```python
from build123d import *

# Parameters (mm, degrees)
SKETCH_1_W               = 72
SKETCH_1_H               = 100
EXTRUDE_1_DEPTH          = 5
SKETCH_2_W               = 72
SKETCH_2_H               = 5
EXTRUDE_2_DEPTH          = 24
CUT_EXTRUDE_1_DEPTH      = 83.443920334
CUT_EXTRUDE_1_DEPTH_BACK = 83.443920334
SKETCH_3_W               = 3
SKETCH_3_H               = 50
CUT_EXTRUDE_2_DEPTH      = 83.443920334
CUT_EXTRUDE_2_DEPTH_BACK = 83.443920334
SKETCH_5_R               = 1.75
CUT_EXTRUDE_3_DEPTH      = 83.443920334
CUT_EXTRUDE_3_DEPTH_BACK = 83.443920334
SKETCH_6_R               = 1.75
CUT_EXTRUDE_4_DEPTH      = 83.443920334
CUT_EXTRUDE_4_DEPTH_BACK = 83.443920334
SKETCH_7_W               = 24
SKETCH_7_H               = 12
FILLET_1_R               = 5
FILLET_2_R               = 2
CUT_EXTRUDE_5_DEPTH      = 83.443920334
CUT_EXTRUDE_5_DEPTH_BACK = 83.443920334
SKETCH_8_R               = 1.75


with BuildPart() as part:
    # 草图1 → 凸台-拉伸1 (new body)
    with BuildSketch(Plane(origin=(0, 0, 0), x_dir=(1, 0, 0), z_dir=(0, 1, 0))):
        Rectangle(SKETCH_1_W, SKETCH_1_H)
    extrude(amount=EXTRUDE_1_DEPTH)

    # 草图2 → 凸台-拉伸2 (add)
    with BuildSketch(Plane.XY.offset(50)):
        with Locations((0, 2.5)):
            Rectangle(SKETCH_2_W, SKETCH_2_H)
    extrude(amount=EXTRUDE_2_DEPTH)

    # 草图3 → 切除-拉伸1 (cut, two sides: drawn at the far end of the back side and taken through both)
    with BuildSketch(Plane(origin=(0, 5, 0), x_dir=(1, 0, 0), z_dir=(0, 1, 0)).offset(-CUT_EXTRUDE_1_DEPTH_BACK)):
        with Locations((-34.5, 25)):
            Rectangle(SKETCH_3_W, SKETCH_3_H)
        with Locations((34.5, 25)):
            Rectangle(SKETCH_3_W, SKETCH_3_H)
        with Locations((-34.5, -49)):
            Rectangle(SKETCH_3_W, SKETCH_3_H)
        with Locations((34.5, -49)):
            Rectangle(SKETCH_3_W, SKETCH_3_H)
    extrude(amount=CUT_EXTRUDE_1_DEPTH + CUT_EXTRUDE_1_DEPTH_BACK, mode=Mode.SUBTRACT)

    # 草图5 → 切除-拉伸2 (cut, two sides: drawn at the far end of the back side and taken through both)
    with BuildSketch(Plane(origin=(0, 5, 0), x_dir=(1, 0, 0), z_dir=(0, 1, 0)).offset(-CUT_EXTRUDE_2_DEPTH_BACK)):
        with Locations(Location((-23.5, 40.5, 0), (0, 0, 270))):
            Circle(SKETCH_5_R)
    extrude(amount=CUT_EXTRUDE_2_DEPTH + CUT_EXTRUDE_2_DEPTH_BACK, mode=Mode.SUBTRACT)

    # 草图6 → 切除-拉伸3 (cut, two sides: drawn at the far end of the back side and taken through both)
    with BuildSketch(Plane(origin=(0, 5, 0), x_dir=(1, 0, 0), z_dir=(0, 1, 0)).offset(-CUT_EXTRUDE_3_DEPTH_BACK)):
        with Locations(Location((23.5, 40.5, 0), (0, 0, 270))):
            Circle(SKETCH_6_R)
        with Locations(Location((-23.5, -64.5, 0), (0, 0, 270))):
            Circle(SKETCH_6_R)
        with Locations(Location((23.5, -64.5, 0), (0, 0, 270))):
            Circle(SKETCH_6_R)
    extrude(amount=CUT_EXTRUDE_3_DEPTH + CUT_EXTRUDE_3_DEPTH_BACK, mode=Mode.SUBTRACT)

    # 草图7 → 切除-拉伸4 (cut, two sides: drawn at the far end of the back side and taken through both)
    with BuildSketch(Plane(origin=(0, 5, 0), x_dir=(1, 0, 0), z_dir=(0, 1, 0)).offset(-CUT_EXTRUDE_4_DEPTH_BACK)):
        with Locations((0, -50)):
            Rectangle(SKETCH_7_W, SKETCH_7_H)
        with Locations((0, 26)):
            Rectangle(SKETCH_7_W, SKETCH_7_H)
    extrude(amount=CUT_EXTRUDE_4_DEPTH + CUT_EXTRUDE_4_DEPTH_BACK, mode=Mode.SUBTRACT)

    # 圆角1
    fillet_1_edges = [part.edges().sort_by_distance(p)[0] for p in [
        (33, 2.5, -50),
        (-33, 2.5, 74),
        (33, 2.5, 74),
        (-33, 2.5, -50),
    ]]
    fillet(fillet_1_edges, radius=FILLET_1_R)

    # 圆角2
    fillet_2_edges = [part.edges().sort_by_distance(p)[0] for p in [
        (36, 2.5, 0),
        (-36, 2.5, 24),
        (36, 2.5, 24),
        (-36, 2.5, 0),
    ]]
    fillet(fillet_2_edges, radius=FILLET_2_R)

    # 草图8 → 切除-拉伸5 (cut, two sides: drawn at the far end of the back side and taken through both)
    with BuildSketch(Plane(origin=(0, 5, 0), x_dir=(1, 0, 0), z_dir=(0, 1, 0)).offset(-CUT_EXTRUDE_5_DEPTH_BACK)):
        with Locations(Location((0, 40.5, 0), (0, 0, 270))):
            Circle(SKETCH_8_R)
        with Locations(Location((0, -64.5, 0), (0, 0, 270))):
            Circle(SKETCH_8_R)
    extrude(amount=CUT_EXTRUDE_5_DEPTH + CUT_EXTRUDE_5_DEPTH_BACK, mode=Mode.SUBTRACT)


solid = part.part
```
The listing builds one solid part. Answer for the finished solid, in the listing's coordinates (mm). A direction names the side the tool comes from. Round coordinates to 2 decimals unless told otherwise and drop trailing zeros. Write each loop counter-clockwise with the first axis right and the second up, starting at its lowest first coordinate (ties: lowest second). Pieces come first, ordered by that corner, then holes. Notation, with made-up numbers: (15, 4) -> (55, 4) arc R21 cw to (55, 32) -> close; hole circle Ø4 at (69.25, -28). An arc over 180 degrees is marked (long way). Answer as a JSON object with one key per item and string values. Group by question number.
Q1. Straight lines are drawn through the part: line 1 along Z through (x, y) = (0, 2.85); line 2 along Z through (x, y) = (10, 1.2); line 3 along X through (y, z) = (3.7, -40.5). For each, find the intervals that lie inside material, in ascending order.
Q2. Section A-A (x = -23.5) is taken. Write down the section's boundary in (y, z), plus the area to 3 significant figures.
Q3. Which of the six approach directions +Z, -Z, +X, -X, +Y, -Y give full straight-line access (tool end or side, diameter ignored) to faces 5 (the face through (12, 2, 50)), 6 (the face through (-33, 2, 47)), 7 (the face through (-33, 2, -22)), 8 (the face through (33, 2, 47))?
Q4. Section B-B (y = 1.2) is taken. Count the separate pieces of the cut face and the enclosed holes in it, plus the area to 3 significant figures.
Q5. Each of these flat-tipped pins is pushed along its axis until it touches: pin 1 Ø1.5 at (y, z) = (2.5, -20.5) entering from +X; pin 2 Ø0.5 at (x, y) = (33.5, 3.5) entering from +Z; pin 3 Ø0.5 at (x, y) = (-33.5, 3.5) entering from -Z; pin 4 Ø2 at (x, z) = (-23.5, -40.5) entering from -Y. Where does it stop, or does it pass through?
Q6. Section C-C (x = 0) is taken. Write down the section's boundary in (y, z), plus the area to 3 significant figures.
Q7. Section D-D (z = -24.5) is taken. Write down the section's boundary in (x, y).
Q8. Determine the mould class of faces 1 (the face through (36, 2, 12)), 2 (the face through (-32, 3, 72)), 3 (the face through (0, 2, -20)), 4 (the face through (31, 3, -49)) for opening direction Z: pulls with the +Z half, pulls with the -Z half, needs draft (parallel to the pull), parting line crosses it, or undercut.
Check values:
{
 "1": {"line 1": "-50 to -42.25, -38.75 to -32, -20 to 44, 56 to 62.75, 66.25 to 74", "line 2": "-50 to -32, -20 to 44, 56 to 74", "line 3": "-33 to -25.25, -21.75 to -1.75, 1.75 to 21.75, 25.25 to 33"},
 "2": {"outline": "(0, -50) -> (5, -50) -> (5, -42.25) -> (0, -42.25) -> close; (0, -38.75) -> (5, -38.75) -> (5, 62.75) -> (0, 62.75) -> close; (0, 66.25) -> (5, 66.25) -> (5, 74) -> (0, 74) -> close", "area": "585 mm^2"},
 "3": {"face 5": "+Y, -Y", "face 6": "+Z, -X, +Y, -Y", "face 7": "-Z, -X, +Y, -Y", "face 8": "+Z, +X, +Y, -Y"},
 "4": {"separate pieces": "1", "enclosed holes": "8", "area": "7,670 mm^2"},
 "5": {"pin 1": "x = 33", "pin 2": "z = 24", "pin 3": "z = 0", "pin 4": "through"},
 "6": {"outline": "(0, -50) -> (5, -50) -> (5, -42.25) -> (0, -42.25) -> close; (0, -38.75) -> (5, -38.75) -> (5, -32) -> (0, -32) -> close; (0, -20) -> (5, -20) -> (5, 44) -> (0, 44) -> close; (0, 56) -> (5, 56) -> (5, 62.75) -> (0, 62.75) -> close; (0, 66.25) -> (5, 66.25) -> (5, 74) -> (0, 74) -> close", "area": "465 mm^2"},
 "7": {"outline": "(-33, 0) -> (-12, 0) -> (-12, 5) -> (-33, 5) -> close; (12, 0) -> (33, 0) -> (33, 5) -> (12, 5) -> close"},
 "8": {"face 1": "needs draft", "face 2": "pulls with the +Z half", "face 3": "undercut", "face 4": "pulls with the -Z half"}
}
